Design review of the part built by this model. Coordinates are the model's own, in mm. Round coordinates to 2 decimals unless told otherwise and drop trailing zeros. Loops run counter-clockwise (first coordinate to the right, second up) from the corner with the lowest first, then second, coordinate; pieces in that order, holes last. Notation, with made-up numbers: (-25, 77) -> (-8, 77) arc R26 cw to (-8, 108) -> close; hole circle Ø11 at (-20.5, 44). An arc over 180 degrees is marked (long way). Use a Markdown table: item, result. Add a question column.
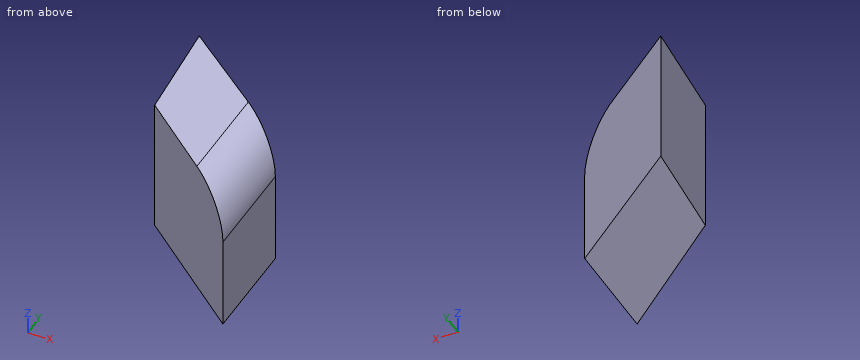
from build123d import *

# Parameters (mm, degrees)
F1_DEPTH = 53
F2_R     = 16.899495


with BuildPart() as f1:
    # F0 (on Top) → F1 (new body)
    with BuildSketch(Plane.XY):
        Polygon((-96.82814, 22.496663), (-93.590319, -16.897356), (-49.226902, -52.804068), (-49.226902, -13.874024), align=None)
    extrude(amount=F1_DEPTH)

    # F2
    f2_edges = [f1.edges().sort_by_distance(p)[0] for p in [
        (-49.226902, -33.339046, 53),
    ]]
    fillet(f2_edges, radius=F2_R)


solid = f1.part
1. Insertion check: P1, Ø5, axis at y = 5.5, z = 35.5, coming from the -X side; P2, Ø4, axis at x = -78, z = 41.5, coming from the +Y side; P3, Ø6, axis at x = -87.5, z = 10.5, coming from the -Y side; P4, Ø6, axis at x = -76, y = -23.5, coming from the -Z side. Each pin has a flat end and moves straight along its axis. Give the tip position at first contact, or say it passes through.
2. Consider section D-D on y = -20. State the section outline as (x, z) points, plus the area to 3 significant figures.
3. Consider section B-B on y = -37.5. State the section outline as (x, z) points.
4. Consider section C-C on x = -78.5. State the section outline as (y, z) points.
5. To check wall thickness, follow probe 1 along Z at (x, y) = (-66, -10); probe 2 along Y at (x, z) = (-83.5, 29.5); probe 3 along X at (y, z) = (11.5, 24). State the ranges of each line that lie inside material, in increasing order. Write a range as from..to.
6. Consider section A-A on z = 14.5. State the section outline as (x, y) points, plus the area to 3 significant figures.
Verdict:
| question | item | result |
|---|---|---|
| 1 | P1 | stops at x = -95.64 |
| 1 | P2 | stops at y = 9.64 |
| 1 | P3 | stops at y = -24.25 |
| 1 | P4 | stops at z = 0 |
| 2 | outline | (-89.76, 0) -> (-49.23, 0) -> (-49.23, 36.1) arc R16.9 ccw to (-66.13, 53) -> (-89.76, 53) -> close |
| 2 | area | 2,090 mm² |
| 3 | outline | (-68.14, 0) -> (-49.23, 0) -> (-49.23, 36.1) arc R16.9 ccw to (-66.13, 53) -> (-68.14, 53) -> close |
| 4 | outline | (-29.11, 0) -> (8.49, 0) -> (8.49, 53) -> (-29.11, 53) -> close |
| 5 | probe 1 | z = 0..53 |
| 5 | probe 2 | y = -25.06..12.31 |
| 5 | probe 3 | x = -95.92..-82.44 |
| 6 | outline | (-96.83, 22.5) -> (-93.59, -16.9) -> (-49.23, -52.8) -> (-49.23, -13.87) -> close |
| 6 | area | 1,740 mm² |
